Build history of the part. All positions in model axes, mm. A direction names the side the tool comes from. Round coordinates to 2 decimals unless told otherwise and drop trailing zeros. Order: outer loops, then holes, each group sorted by start corner. A loop starts at its lowest first (then second) coordinate and runs counter-clockwise, first axis right, second up. Notation, with made-up numbers: (80, 3.5) -> (96, 3.5) arc R26 cw to (96, 38.5) -> close; hole circle Ø3 at (24.25, -3.5). An arc over 180 degrees is marked (long way). Use a Markdown table: item, result. Add a question column.
Item 1: Slice it at A-A, the plane z = 8.25. Give the cut face in (x, y).
Item 2: Two-plate mould, pull along Z, no slides. Class faces 5 (the face through (20, 2, 26.3)), 6 (the face through (23, 0.5, 12.5)), 7 (the face through (29, 4, 0)), 8 (the face through (9, 0.5, 0)): released by +Z, released by -Z, zero draft, split by the parting line, or undercut.
Item 3: Probe L1, parallel to X at y = 3.3, z = 21.5; L2, parallel to Z at x = 38, y = 0.55; L3, parallel to Z at x = 18.5, y = 2.65. List the from-to ranges inside material, lowest first.
Item 4: Pin check, flat tips, straight feed: pin 1 (1.2 mm diameter, centred on y = 2, z = 2, fed in from +X); pin 2 (0.5 mm diameter, centred on x = 40.5, y = 0.5, fed in from +Z); pin 3 (7.5 mm diameter, centred on x = 26, z = 16, fed in from +Y); pin 4 (2 mm diameter, centred on x = 31.5, z = 21.5, fed in from -Y). Stop position of each tip, or through.
Item 5: Slice it at D-D, the plane x = 38.5. Give the cut face in (y, z).
Item 6: Slice it at B-B, the plane x = 20. Give the cut face in (y, z), plus the area to 3 significant figures.
Item 7: 3-axis set-ups, long thin cutter, end or side, ignore diameter. For faces 1 (the face through (41.6, 0.5, 0)), 2 (the face through (25.4, 0.5, 25.3)), 3 (the face through (20.7, 0.5, 12.8)), 4 (the face through (31, 3, 0)): which of +Z, -Z, +X, -X, +Y, -Y reach the whole face in a straight line?
Item 8: Slice it at C-C, the plane y = 1.9. Give the cut face in (x, z).
from build123d import *

# Parameters (mm, degrees)
SKETCH_1_W          = 50.8
SKETCH_1_H          = 25.3
EXTRUDE_1_DEPTH     = 1
SKETCH_3_W          = 1
SKETCH_3_H          = 4
EXTRUDE_3_DEPTH     = 3
SKETCH_4_W          = 4
SKETCH_4_H          = 4
EXTRUDE_5_DEPTH     = 1
SKETCH_5_W          = 4
SKETCH_5_H          = 4
EXTRUDE_6_DEPTH     = 1
SKETCH_6_W          = 8.783145701
SKETCH_6_H          = 22.3
SKETCH_6_W_2        = 7.155556096
SKETCH_6_W_3        = 5.4
CUT_EXTRUDE_1_DEPTH = 58.343962193


with BuildPart() as part:
    # 草图1 → 凸台-拉伸1 (new body)
    with BuildSketch(Plane(origin=(0, 0, 0), x_dir=(1, 0, 0), z_dir=(0, 1, 0))):
        with Locations((25.4, -12.65)):
            Rectangle(SKETCH_1_W, SKETCH_1_H)
    extrude(amount=EXTRUDE_1_DEPTH)

    # 草图3 → 凸台-拉伸3 (add)
    with BuildSketch(Plane(origin=(0, 1, 0), x_dir=(1, 0, 0), z_dir=(0, 1, 0))):
        with Locations((21.7, -23.3)):
            Rectangle(SKETCH_3_W, SKETCH_3_H)
        with Locations((21.7, -2)):
            Rectangle(SKETCH_3_W, SKETCH_3_H)
        with Locations((29.1, -2)):
            Rectangle(SKETCH_3_W, SKETCH_3_H)
        with Locations((29.1, -23.3)):
            Rectangle(SKETCH_3_W, SKETCH_3_H)
    extrude(amount=EXTRUDE_3_DEPTH)

    # 草图4 → 凸台-拉伸5 (add)
    with BuildSketch(Plane.XY.offset(25.3)):
        with Locations((20.2, 2)):
            Rectangle(SKETCH_4_W, SKETCH_4_H)
        with Locations((30.6, 2)):
            Rectangle(SKETCH_4_W, SKETCH_4_H)
    extrude(amount=EXTRUDE_5_DEPTH)

    # 草图5 → 凸台-拉伸6 (add)
    with BuildSketch(Plane(origin=(0, 0, 0), x_dir=(-1, 0, 0), z_dir=(0, 0, -1))):
        with Locations((-20.2, 2)):
            Rectangle(SKETCH_5_W, SKETCH_5_H)
        with Locations((-30.6, 2)):
            Rectangle(SKETCH_5_W, SKETCH_5_H)
    extrude(amount=EXTRUDE_6_DEPTH)

    # 草图6 → 切除-拉伸1 (cut, through all)
    with BuildSketch(Plane.XZ):
        Polygon((20.7, 1.5), (19.7, 1.5), (9.655556096, 1.5), (9.655556096, 23.8), (19.7, 23.8), (20.7, 23.8), align=None)
        Polygon((30.1, 23.8), (31.1, 23.8), (39.516854299, 23.8), (39.516854299, 1.5), (31.1, 1.5), (30.1, 1.5), align=None)
        with Locations((44.908427149, 12.65)):
            Rectangle(SKETCH_6_W, SKETCH_6_H)
        with Locations((5.077778048, 12.65)):
            Rectangle(SKETCH_6_W_2, SKETCH_6_H)
        with Locations((25.7, 12.65)):
            Rectangle(SKETCH_6_W_3, SKETCH_6_H)
    extrude(amount=-CUT_EXTRUDE_1_DEPTH, mode=Mode.SUBTRACT)


solid = part.part
Check sheet entries:
| question | item | result |
|---|---|---|
| 1 | outline | (0, 0) -> (1.5, 0) -> (1.5, 1) -> (0, 1) -> close; (8.66, 0) -> (9.66, 0) -> (9.66, 1) -> (8.66, 1) -> close; (20.7, 0) -> (23, 0) -> (23, 1) -> (20.7, 1) -> close; (28.4, 0) -> (30.1, 0) -> (30.1, 1) -> (28.4, 1) -> close; (39.52, 0) -> (40.52, 0) -> (40.52, 1) -> (39.52, 1) -> close; (49.3, 0) -> (50.8, 0) -> (50.8, 1) -> (49.3, 1) -> close |
| 2 | face 5 | released by +Z |
| 2 | face 6 | undercut |
| 2 | face 7 | zero draft |
| 2 | face 8 | released by -Z |
| 3 | L1 | 21.2 to 22.2, 28.6 to 29.6 |
| 3 | L2 | 0 to 1.5, 23.8 to 25.3 |
| 3 | L3 | -1 to 0, 25.3 to 26.3 |
| 4 | pin 1 | x = 29.6 |
| 4 | pin 2 | z = 25.3 |
| 4 | pin 3 | y = 1 |
| 4 | pin 4 | through |
| 5 | outline | (0, 0) -> (1, 0) -> (1, 1.5) -> (0, 1.5) -> close; (0, 23.8) -> (1, 23.8) -> (1, 25.3) -> (0, 25.3) -> close |
| 6 | outline | (0, -1) -> (4, -1) -> (4, 0) -> (1, 0) -> (1, 1.5) -> (0, 1.5) -> close; (0, 23.8) -> (1, 23.8) -> (1, 25.3) -> (4, 25.3) -> (4, 26.3) -> (0, 26.3) -> close |
| 6 | area | 11.0 mm2 |
| 7 | face 1 | -Z, +X, +Y, -Y |
| 7 | face 2 | +Z, +Y, -Y |
| 7 | face 3 | +Y, -Y |
| 7 | face 4 | +X, +Y |
| 8 | outline | (18.2, -1) -> (22.2, -1) -> (22.2, 4) -> (21.2, 4) -> (21.2, 0) -> (18.2, 0) -> close; (18.2, 25.3) -> (21.2, 25.3) -> (21.2, 21.3) -> (22.2, 21.3) -> (22.2, 26.3) -> (18.2, 26.3) -> close; (28.6, -1) -> (32.6, -1) -> (32.6, 0) -> (29.6, 0) -> (29.6, 4) -> (28.6, 4) -> close; (28.6, 21.3) -> (29.6, 21.3) -> (29.6, 25.3) -> (32.6, 25.3) -> (32.6, 26.3) -> (28.6, 26.3) -> close |
